Part model, mm, in its own coordinate system. A direction names the side the tool comes from. Round coordinates to 2 decimals unless told otherwise and drop trailing zeros. Loops run counter-clockwise (first coordinate to the right, second up) from the corner with the lowest first, then second, coordinate; pieces in that order, holes last. Notation, with made-up numbers: (48.5, 85.5) -> (65.5, 85.5) arc R24 ccw to (65.5, 105.5) -> close; hole circle Ø7 at (88, 36). An arc over 180 degrees is marked (long way). Answer as CSV lines item,"result".
from build123d import *

# Parameters (mm, degrees)
BOSS_EXTRUDE1_DEPTH = 5
SKETCH2_R           = 1.5
SKETCH2_W           = 10
SKETCH2_H           = 5
CUT_EXTRUDE1_DEPTH  = 10
FILLET1_R           = 10
FILLET2_R           = 1
CONG_1_R            = 1


with BuildPart() as part:
    # Sketch1 → Boss-Extrude1 (new body)
    with BuildSketch(Plane.XY):
        Polygon((-32.518889855, -56.191512275), (-30.018889855, -56.191512275), (-30.018889855, -61.191512275), (-20.018889855, -61.191512275), (-20.018889855, -56.191512275), (-11.518889855, -56.191512275), (-11.518889855, -53.191512275), (-12.618889855, -53.191512275), (-12.618889855, -50.891512275), (-11.518889855, -50.891512275), (-11.518889855, -46.191512275), (-8.518889855, -46.191512275), (-8.518889855, -50.891512275), (-7.418889855, -50.891512275), (-7.418889855, -53.191512275), (-8.518889855, -53.191512275), (-8.518889855, -56.191512275), (-0.018889855, -56.191512275), (-0.018889855, -61.191512275), (9.981110145, -61.191512275), (9.981110145, -56.191512275), (12.481110145, -56.191512275), (12.481110145, -61.191512275), (40.481110145, -61.191512275), (12.481110145, -16.103821473), (12.481110145, 58.808487725), (9.981110145, 58.808487725), (9.981110145, 68.808487725), (-0.018889855, 68.808487725), (-0.018889855, 58.808487725), (-8.518889855, 58.808487725), (-8.518889855, 50.808487725), (-7.418889855, 50.808487725), (-7.418889855, 48.508487725), (-8.518889855, 48.508487725), (-8.518889855, 43.808487725), (-11.518889855, 43.808487725), (-11.518889855, 48.508487725), (-12.618889855, 48.508487725), (-12.618889855, 50.808487725), (-11.518889855, 50.808487725), (-11.518889855, 58.808487725), (-20.018889855, 58.808487725), (-20.018889855, 68.808487725), (-30.018889855, 68.808487725), (-30.018889855, 58.808487725), (-32.518889855, 58.808487725), (-32.518889855, -16.103821473), (-60.518889855, -61.191512275), (-32.518889855, -61.191512275), align=None)
    extrude(amount=BOSS_EXTRUDE1_DEPTH)

    # Sketch2 → Cut-Extrude1 (cut)
    with BuildSketch(Plane.XY.offset(5)):
        with Locations((-10.018889855, 16.308487725)):
            Circle(SKETCH2_R)
        with Locations((-25.018889855, 16.308487725)):
            Rectangle(SKETCH2_W, SKETCH2_H)
        with Locations((4.981110145, 16.308487725)):
            Rectangle(SKETCH2_W, SKETCH2_H)
    extrude(amount=-CUT_EXTRUDE1_DEPTH, mode=Mode.SUBTRACT)

    # Fillet1
    fillet1_edges = [part.edges().sort_by_distance(p)[0] for p in [
        (-32.518889855, -16.103821473, 2.5),
        (12.481110145, -16.103821473, 2.5),
    ]]
    fillet(fillet1_edges, radius=FILLET1_R)

    # Fillet2
    fillet2_edges = [part.edges().sort_by_distance(p)[0] for p in [
        (40.481110145, -61.191512275, 2.5),
        (-60.518889855, -61.191512275, 2.5),
    ]]
    fillet(fillet2_edges, radius=FILLET2_R)

    # Congé1
    cong_1_edges = [part.edges().sort_by_distance(p)[0] for p in [
        (-30.018889855, 68.808487725, 2.5),
        (-20.018889855, 68.808487725, 2.5),
        (-0.018889855, 68.808487725, 2.5),
        (9.981110145, 68.808487725, 2.5),
    ]]
    fillet(cong_1_edges, radius=CONG_1_R)


solid = part.part
Q1. Drill centre lines: line 1 along X through (y, z) = (17, 0.5); line 2 along X through (y, z) = (62, 2.8); line 3 along Y through (x, z) = (-14.5, 1.8). Where is each one in solid material? Low to high.
Geometry results:
line 1,"-32.52 to -30.02, -20.02 to -11.35, -8.69 to -0.02, 9.98 to 12.48"
line 2,"-30.02 to -20.02, -0.02 to 9.98"
line 3,"-56.19 to 58.81"
Q2. Drop flat-ended pins along their axis: P1, Ø2.5, axis at y = -48.5, z = 3.5, coming from the +X side; P2, Ø0.9, axis at y = -55, z = 2.5, coming from the +X side; P3, Ø0.5, axis at x = -8, z = 3, coming from the -Y side. Give the stop position or say it passes through.
Geometry results:
P1,"x = 33.38"
P2,"x = 36.92"
P3,"y = -56.19"
Q3. Saw through at B-B, the plane y = -3. Write the cut outline in (x, z).
Geometry results:
outline,"(-32.52, 0) -> (12.48, 0) -> (12.48, 5) -> (-32.52, 5) -> close"
Q4. Which spindle directions (+Z, -Z, +X, -X, +Y, -Y) get a long thin tool onto all of the face, cutting with end or side? Do faces 1 (the face through (-11.519, -49, 2)), 2 (the face through (-10, 43.808, 2)), 3 (the face through (-25, 13.808, 3)). Say none if no direction does.
Geometry results:
face 1,"+Z, -Z, -Y"
face 2,"+Z, -Z, +Y"
face 3,"+Z, -Z"
Q5. Two-plate mould, pull along X, no slides. Class faces 4 (the face through (-25, 18.808, 3)), 5 (the face through (9.981, 63, 2)), 6 (the face through (-46.62, -38.81, 2.46)): pulls with the +X half, pulls with the -X half, needs draft (parallel to the pull), parting line crosses it, or undercut.
Geometry results:
face 4,"undercut"
face 5,"pulls with the +X half"
face 6,"pulls with the -X half"
Q6. Saw through at C-C, the plane z = 2.7. Give the number of separate pieces and of enclosed holes in the cut face, then the cut area to 3 significant figures.
Geometry results:
separate pieces,"1"
enclosed holes,"3"
area,"6,540 mm2"
Q7. Saw through at A-A, the plane x = 2.5. Write the cut outline in (y, z).
Geometry results:
outline,"(-61.19, 0) -> (13.81, 0) -> (13.81, 5) -> (-61.19, 5) -> close; (18.81, 0) -> (68.81, 0) -> (68.81, 5) -> (18.81, 5) -> close"
Q8. Saw through at D-D, the plane x = 19. Write the cut outline in (y, z), then the cut area to 3 significant figures.
Geometry results:
outline,"(-61.19, 0) -> (-26.6, 0) -> (-26.6, 5) -> (-61.19, 5) -> close"
area,"173 mm2"
